Verification items for the finished model (mm, model axes). A direction names the side the tool comes from. Round coordinates to 2 decimals unless told otherwise and drop trailing zeros. Write each loop counter-clockwise with the first axis right and the second up, starting at its lowest first coordinate (ties: lowest second). Pieces come first, ordered by that corner, then holes. Notation, with made-up numbers: (83.25, 9) - (114.25, 9) arc R24 ccw to (114.25, 33) - close; hole circle Ø1 at (35.5, -21). An arc over 180 degrees is marked (long way). Answer as a JSON object with one key per item and string values. Group by question number.
1) Section check A-A (x = -16). Enter the section's corners in (y, z) (1 decimal), then the cut area to 3 significant figures.
2) Set-up check for faces 4 (the flat face through (11.8, 14.655, 42.08)), 5 (the flat face through (-9.525, 0, 17)), 6 (the flat face through (11.334, 7.372, 42.08)), 7 (the flat face through (9.525, 0, 17)): record each of +Z, -Z, +X, -X, +Y, -Y from which the full face is reachable in a straight line by a thin tool's end or side.
3) Mould release check, pull along Z, two halves, no side actions. Record for faces 1 (the cylindrical face through (-18.473, 11.223, 42.08)), 2 (the cylindrical face through (-1.377, 4.914, 35.708)), 3 (the flat face through (0, 11, 42.863)): +Z half, -Z half, draft (parallel to the pull), parting line (faces both ways), or undercut.
4) Section check D-D (y = 1). Enter the section's corners in (x, z) (3 decimals), then the cut area to 3 significant figures.
5) Section check C-C (z = 31). Enter the section's corners in (x, y) (3 decimals), then the cut area to 3 significant figures.
6) Thickness scan on line 1 (Z direction, x = 3, y = 15.5) (1 decimal); line 2 (X direction, y = -3.5, z = 16) (3 decimals); line 3 (Z direction, x = 3, y = -6) (3 decimals). Record the ranges inside material, lowest first.
7) Go/stop test with flat-tipped pins: pin 1 Ø3 at (x, z) = (-4.5, 36.5) entering from +Y; pin 2 Ø1 at (x, y) = (12.86, 11.53) entering from -Z; pin 3 Ø1.8 at (x, y) = (16.03, 11.53) entering from -Z (3 decimals); pin 4 Ø10 at (y, z) = (-12, 32) entering from -X (3 decimals). Record where each tip stops, or that it passes through.
```python
from build123d import *

# Parameters (mm, degrees)
SKETCH1_W               = 19.05
SKETCH1_H               = 38.1
BOSS_EXTRUDE1_DEPTH     = 34.925
SKETCH2_R               = 6.35
BOSS_EXTRUDE2_DEPTH     = 1.5875
SKETCH3_R               = 4.7625
BOSS_EXTRUDE3_DEPTH     = 6.35
BOSS_EXTRUDE4_DEPTH     = 1.5875
SKETCH5_R               = 0.79375
CUT_EXTRUDE1_DEPTH      = 6.35
LPATTERN1_COUNT         = 5
LPATTERN1_PITCH         = 3.175
MIRROR1_COPY_1_SKETCH_R = 0.79375
MIRROR1_COPY_1_DEPTH    = 6.35
MIRROR1_COPY_2_SKETCH_R = 0.79375
MIRROR1_COPY_2_DEPTH    = 6.35
MIRROR1_COPY_3_SKETCH_R = 0.79375
MIRROR1_COPY_3_DEPTH    = 6.35
MIRROR1_COPY_4_SKETCH_R = 0.79375
MIRROR1_COPY_4_DEPTH    = 6.35


with BuildPart() as part:
    # Sketch1 → Boss-Extrude1 (new body)
    with BuildSketch(Plane.XY):
        Rectangle(SKETCH1_W, SKETCH1_H)
    extrude(amount=BOSS_EXTRUDE1_DEPTH)

    # Sketch2 → Boss-Extrude2 (add)
    with BuildSketch(Plane.XY.offset(34.925)):
        with Locations((0, 11.1125)):
            Circle(SKETCH2_R)
    extrude(amount=BOSS_EXTRUDE2_DEPTH)

    # Sketch3 → Boss-Extrude3 (add)
    with BuildSketch(Plane.XY.offset(36.5125)):
        with Locations((0, 11.30801151)):
            Circle(SKETCH3_R)
    extrude(amount=BOSS_EXTRUDE3_DEPTH)

    # Sketch4 → Boss-Extrude4 (add)
    with BuildSketch(Plane.XY.offset(42.8625)):
        with BuildLine():
            Line((0, 16.07051151), (-22.253587721, 14.127262895))
            ThreePointArc((-22.253587721, 14.127262895), (-24.76292538, 11.561183994), (-22.197271079, 9.051412208))
            Line((-22.197271079, 9.051412208), (0, 6.54551151))
            Line((0, 6.54551151), (22.279071817, 8.170731681))
            ThreePointArc((22.279071817, 8.170731681), (24.844676693, 10.840221296), (22.179280362, 13.410078409))
            Line((22.179280362, 13.410078409), (0, 16.07051151))
        make_face()
    extrude(amount=-BOSS_EXTRUDE4_DEPTH)

    # Sketch5 → Cut-Extrude1 (cut)
    with BuildSketch(Plane.XY.offset(42.8625)):
        with Locations((-22.38167538, 11.526576548)):
            Circle(SKETCH5_R)
    cut_extrude1 = extrude(amount=-CUT_EXTRUDE1_DEPTH, mode=Mode.SUBTRACT)

    # LPattern1: Cut-Extrude1 ×5
    with Locations(*[(i * LPATTERN1_PITCH, 0, 0) for i in range(1, LPATTERN1_COUNT)]):
        add(cut_extrude1, mode=Mode.SUBTRACT)

    # Mirror1: Cut-Extrude1 across plane
    add(cut_extrude1.mirror(Plane(origin=(0, 0, 0), x_dir=(0, 0, 1), z_dir=(1, 0, 0))), mode=Mode.SUBTRACT)

    # Mirror1 copy 1 sketch → Mirror1 copy 1 (cut)
    with BuildSketch(Plane(origin=(-3.175, 0, 42.8625), x_dir=(-1, 0, 0), z_dir=(0, 0, 1))):
        with Locations((-22.38167538, -11.526576548)):
            Circle(MIRROR1_COPY_1_SKETCH_R)
    extrude(amount=-MIRROR1_COPY_1_DEPTH, mode=Mode.SUBTRACT)

    # Mirror1 copy 2 sketch → Mirror1 copy 2 (cut)
    with BuildSketch(Plane(origin=(-6.35, 0, 42.8625), x_dir=(-1, 0, 0), z_dir=(0, 0, 1))):
        with Locations((-22.38167538, -11.526576548)):
            Circle(MIRROR1_COPY_2_SKETCH_R)
    extrude(amount=-MIRROR1_COPY_2_DEPTH, mode=Mode.SUBTRACT)

    # Mirror1 copy 3 sketch → Mirror1 copy 3 (cut)
    with BuildSketch(Plane(origin=(-9.525, 0, 42.8625), x_dir=(-1, 0, 0), z_dir=(0, 0, 1))):
        with Locations((-22.38167538, -11.526576548)):
            Circle(MIRROR1_COPY_3_SKETCH_R)
    extrude(amount=-MIRROR1_COPY_3_DEPTH, mode=Mode.SUBTRACT)

    # Mirror1 copy 4 sketch → Mirror1 copy 4 (cut)
    with BuildSketch(Plane(origin=(-12.7, 0, 42.8625), x_dir=(-1, 0, 0), z_dir=(0, 0, 1))):
        with Locations((-22.38167538, -11.526576548)):
            Circle(MIRROR1_COPY_4_SKETCH_R)
    extrude(amount=-MIRROR1_COPY_4_DEPTH, mode=Mode.SUBTRACT)


solid = part.part
```
Returned:
{
 "1": {"outline": "(8.4, 41.3) - (10.7, 41.3) - (10.7, 42.9) - (8.4, 42.9) - close; (12.3, 41.3) - (14.7, 41.3) - (14.7, 42.9) - (12.3, 42.9) - close", "area": "7.52 mm2"},
 "2": {"face 4": "+Z, +X, +Y", "face 5": "-Z, -X, +Y, -Y", "face 6": "+Z, +X, -Y", "face 7": "-Z, +X, +Y, -Y"},
 "3": {"face 1": "draft", "face 2": "undercut", "face 3": "+Z half"},
 "4": {"outline": "(-9.525, 0) - (9.525, 0) - (9.525, 34.925) - (-9.525, 34.925) - close", "area": "665 mm2"},
 "5": {"outline": "(-9.525, -19.05) - (9.525, -19.05) - (9.525, 19.05) - (-9.525, 19.05) - close", "area": "726 mm2"},
 "6": {"line 1": "0 to 36.5, 41.3 to 42.9", "line 2": "-9.525 to 9.525", "line 3": "0 to 34.925"},
 "7": {"pin 1": "y = 16.71", "pin 2": "through", "pin 3": "z = 41.275", "pin 4": "x = -9.525"}
}
